Check sheet for the modelled part. Datum: model origin and axes. Units: mm. Face numbers are marked on the shaded views. A direction names the side the tool comes from. Coordinates: 2 decimals unless noted, no trailing zeros. Write each loop counter-clockwise with the first axis right and the second up, starting at its lowest first coordinate (ties: lowest second). Pieces come first, ordered by that corner, then holes. Notation, with made-up numbers: (-1, 5) -> (27, 5) arc R35 ccw to (27, 39) -> close; hole circle Ø9 at (13.25, 87). An arc over 180 degrees is marked (long way). Put each result on its own line as item: value.
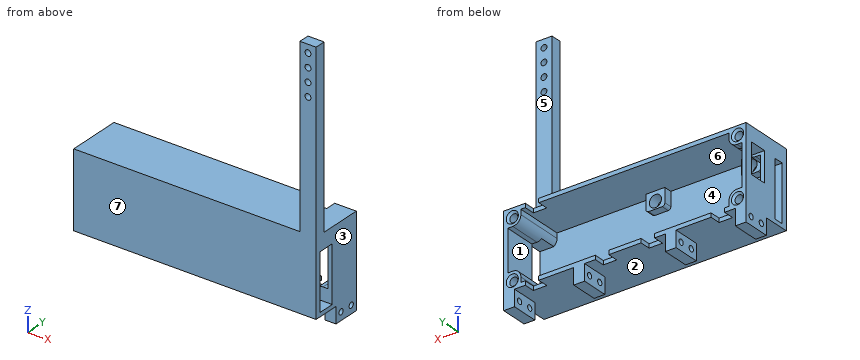
```python
from build123d import *

# Parameters (mm, degrees)
SKETCH2_W           = 87
SKETCH2_H           = 25
BOSS_EXTRUDE1_DEPTH = 2
SKETCH2_3_W         = 90
SKETCH2_3_H         = 28
SKETCH2_3_W_2       = 87
SKETCH2_3_H_2       = 25
BOSS_EXTRUDE2_DEPTH = 20
SKETCH3_W           = 4
SKETCH3_H           = 10.1
BOSS_EXTRUDE3_DEPTH = 6
SKETCH5_R           = 1.05
CUT_EXTRUDE2_DEPTH  = 105
SKETCH3_5_W         = 5
SKETCH3_5_H         = 4
CUT_EXTRUDE3_DEPTH  = 16
SKETCH2_4_W         = 6
SKETCH2_4_H         = 55
BOSS_EXTRUDE4_DEPTH = 4
SKETCH8_W           = 4.863961031
SKETCH8_H           = 4.863961031
SKETCH8_W_2         = 4.86396103
BOSS_EXTRUDE5_DEPTH = 18
SKETCH9_R           = 1.5
CUT_EXTRUDE6_DEPTH  = 5
SKETCH6_W           = 11.14966652
SKETCH6_H           = 6.5
CUT_EXTRUDE4_DEPTH  = 16
FILLET1_R           = 3
SKETCH10_W          = 20.745878282
SKETCH10_H          = 3.532229036
CUT_EXTRUDE7_DEPTH  = 109.1
SKETCH11_W          = 5
SKETCH11_H          = 4
CUT_EXTRUDE8_DEPTH  = 4
SKETCH12_W          = 20.745878282
SKETCH12_H          = 2.501759487
CUT_EXTRUDE10_DEPTH = 8
SKETCH13_R          = 2.25
BOSS_EXTRUDE6_DEPTH = 3
CHAMFER1_SIZE       = 0.75
SKETCH17_W          = 6
SKETCH17_H          = 4
BOSS_EXTRUDE9_DEPTH = 10
SKETCH7_R           = 1.1
CUT_EXTRUDE5_DEPTH  = 10
CUT_EXTRUDE11_START = -1
SKETCH18_R          = 2.25
CUT_EXTRUDE11_DEPTH = 1


with BuildPart() as part:
    # Sketch2 → Boss-Extrude1 (new body)
    with BuildSketch(Plane(origin=(0, 0, 0), x_dir=(1, 0, 0), z_dir=(0, 1, 0))):
        with Locations((-2.329700272, 12.5)):
            Rectangle(SKETCH2_W, SKETCH2_H)
    extrude(amount=BOSS_EXTRUDE1_DEPTH)

    # Sketch2<3> → Boss-Extrude2 (add)
    with BuildSketch(Plane(origin=(0, 0, 0), x_dir=(1, 0, 0), z_dir=(0, 1, 0))):
        with Locations((-2.329700272, 12.5)):
            Rectangle(SKETCH2_3_W, SKETCH2_3_H)
        with Locations((-2.329700272, 12.5)):
            Rectangle(SKETCH2_3_W_2, SKETCH2_3_H_2, mode=Mode.SUBTRACT)
    extrude(amount=BOSS_EXTRUDE2_DEPTH)

    # Sketch3 → Boss-Extrude3 (add)
    with BuildSketch(Plane(origin=(0, 0, -26.5), x_dir=(-1, 0, 0), z_dir=(0, 0, -1))):
        with Locations((45.329700272, 14.95)):
            Rectangle(SKETCH3_W, SKETCH3_H)
        with Locations((-14.670299728, 14.95)):
            Rectangle(SKETCH3_W, SKETCH3_H)
        with Locations((-40.670299728, 14.95)):
            Rectangle(SKETCH3_W, SKETCH3_H)
        with Locations((19.329700272, 14.95)):
            Rectangle(SKETCH3_W, SKETCH3_H)
    extrude(amount=BOSS_EXTRUDE3_DEPTH)

    # Sketch5 → Cut-Extrude2 (cut)
    with BuildSketch(Plane.ZY.offset(47.329700272)):
        with Locations((-29.5, 12.425)):
            Circle(SKETCH5_R)
        with Locations((-29.5, 17.475)):
            Circle(SKETCH5_R)
    extrude(amount=-CUT_EXTRUDE2_DEPTH, mode=Mode.SUBTRACT)

    # Sketch3<5> → Cut-Extrude3 (cut)
    with BuildSketch(Plane(origin=(0, 0, -26.5), x_dir=(-1, 0, 0), z_dir=(0, 0, -1))):
        with Locations((36.829700272, 18)):
            Rectangle(SKETCH3_5_W, SKETCH3_5_H)
        with Locations((10.829700272, 18)):
            Rectangle(SKETCH3_5_W, SKETCH3_5_H)
        with Locations((-32.170299728, 18)):
            Rectangle(SKETCH3_5_W, SKETCH3_5_H)
        with Locations((-6.170299728, 18)):
            Rectangle(SKETCH3_5_W, SKETCH3_5_H)
    extrude(amount=-CUT_EXTRUDE3_DEPTH, mode=Mode.SUBTRACT)

    # Sketch2<4> → Boss-Extrude4 (add)
    with BuildSketch(Plane(origin=(0, 0, 0), x_dir=(1, 0, 0), z_dir=(0, 1, 0))):
        with Locations((39.670299728, -29)):
            Rectangle(SKETCH2_4_W, SKETCH2_4_H)
    extrude(amount=BOSS_EXTRUDE4_DEPTH)

    # Sketch8 → Boss-Extrude5 (add)
    with BuildSketch(Plane(origin=(0, 2, 0), x_dir=(1, 0, 0), z_dir=(0, 1, 0))):
        with Locations((38.738319213, 22.568019484)):
            Rectangle(SKETCH8_W, SKETCH8_H)
        with Locations((38.738319213, 2.431980516)):
            Rectangle(SKETCH8_W, SKETCH8_H)
        with Locations((-43.397719757, 22.568019484)):
            Rectangle(SKETCH8_W_2, SKETCH8_H)
        with Locations((-43.397719757, 2.431980516)):
            Rectangle(SKETCH8_W_2, SKETCH8_H)
    extrude(amount=BOSS_EXTRUDE5_DEPTH)

    # Sketch9 → Cut-Extrude6 (cut)
    with BuildSketch(Plane(origin=(0, 20, 0), x_dir=(1, 0, 0), z_dir=(0, 1, 0))):
        with Locations(Location((-44.147719757, 23.318019485, 0), (0, 0, 270))):
            Circle(SKETCH9_R)
        with Locations(Location((-44.147719757, 1.681980515, 0), (0, 0, 90))):
            Circle(SKETCH9_R)
        with Locations(Location((39.488319212, 1.681980515, 0), (0, 0, 270))):
            Circle(SKETCH9_R)
        with Locations(Location((39.488319212, 23.318019485, 0), (0, 0, 90))):
            Circle(SKETCH9_R)
    extrude(amount=-CUT_EXTRUDE6_DEPTH, mode=Mode.SUBTRACT)

    # Sketch6 → Cut-Extrude4 (cut)
    with BuildSketch(Plane.ZY.offset(47.329700272)):
        with Locations((-9.5, 14)):
            Rectangle(SKETCH6_W, SKETCH6_H)
    extrude(amount=-CUT_EXTRUDE4_DEPTH, mode=Mode.SUBTRACT)

    # Fillet1
    # the kernel refuses this fillet: 3 mm, written as the material it takes off along each edge
    with BuildSketch(Plane(origin=(36.306338697, 2, -4.863961031), x_dir=(0, 0, 1), z_dir=(0, 1, 0)), Plane(origin=(-40.965739242, 2, -20.136038969), x_dir=(0, 0, -1), z_dir=(0, 1, 0))) as fillet1_piece_1:
        with BuildLine():
            CenterArc((FILLET1_R, FILLET1_R), FILLET1_R, 180, 90)
            Line((0, FILLET1_R), (0, 0))
            Line((0, 0), (FILLET1_R, 0))
        make_face()
    extrude(amount=25.5, mode=Mode.SUBTRACT)
    with BuildSketch(Plane(origin=(36.306338697, 2, -20.136038969), x_dir=(0, 0, -1), z_dir=(0, 1, 0))) as fillet1_piece_2:
        with BuildLine():
            CenterArc((FILLET1_R, -FILLET1_R), FILLET1_R, 90, 90)
            Line((0, -FILLET1_R), (0, 0))
            Line((0, 0), (FILLET1_R, 0))
        make_face()
    extrude(amount=25.5, mode=Mode.SUBTRACT)
    with BuildSketch(Plane(origin=(-40.965739242, 2, -4.863961031), x_dir=(0, 0, 1), z_dir=(0, 1, 0))) as fillet1_piece_3:
        with BuildLine():
            CenterArc((FILLET1_R, -FILLET1_R), FILLET1_R, 90, 90)
            Line((0, -FILLET1_R), (0, 0))
            Line((0, 0), (FILLET1_R, 0))
        make_face()
    extrude(amount=16.25, mode=Mode.SUBTRACT)
    with BuildSketch(Plane(origin=(-40.965739242, 9.75, -4.863961031), x_dir=(-1, 0, 0), z_dir=(0, 1, 0))) as fillet1_piece_4:
        with BuildLine():
            CenterArc((FILLET1_R, FILLET1_R), FILLET1_R, 180, 90)
            Line((0, FILLET1_R), (0, 0))
            Line((0, 0), (FILLET1_R, 0))
        make_face()
    extrude(amount=17.75, mode=Mode.SUBTRACT)

    # Sketch10 → Cut-Extrude7 (cut)
    with BuildSketch(Plane.ZY.offset(47.329700272)):
        with Locations((-14.627060859, 3.766114518)):
            Rectangle(SKETCH10_W, SKETCH10_H)
    extrude(amount=-CUT_EXTRUDE7_DEPTH, mode=Mode.SUBTRACT)

    # Sketch11 → Cut-Extrude8 (cut)
    with BuildSketch(Plane.XY.offset(1.5)):
        with Locations((32.170299728, 18)):
            Rectangle(SKETCH11_W, SKETCH11_H)
    extrude(amount=-CUT_EXTRUDE8_DEPTH, mode=Mode.SUBTRACT)

    # Sketch12 → Cut-Extrude10 (cut)
    with BuildSketch(Plane(origin=(42.670299728, 0, 0), x_dir=(0, 0, -1), z_dir=(1, 0, 0))):
        with Locations((14.627060859, 6.78310878)):
            Rectangle(SKETCH12_W, SKETCH12_H)
    extrude(amount=-CUT_EXTRUDE10_DEPTH, mode=Mode.SUBTRACT)

    # Sketch13 → Boss-Extrude6 (add)
    # profile 1 of 2: a face of its own
    with BuildSketch(Plane(origin=(0, 2, 0), x_dir=(1, 0, 0), z_dir=(0, 1, 0))):
        with BuildLine():
            Line((-40.965739242, 1.863961031), (-40.965739242, 0))
            Line((-40.965739242, 0), (-34.465739242, 0))
            Line((-34.465739242, 0), (-34.465739242, 5.247890406))
            ThreePointArc((-34.465739242, 5.247890406), (-34.758632461, 5.954997187), (-35.465739242, 6.247890406))
            Line((-35.465739242, 6.247890406), (-40.619194745, 6.247890406))
            ThreePointArc((-40.619194745, 6.247890406), (-41.102765854, 6.123195485), (-41.465739242, 5.78020837))
            ThreePointArc((-41.465739242, 5.78020837), (-41.553823791, 5.60351457), (-41.605476886, 5.412958687))
            Line((-41.605476886, 5.412958687), (-41.844418898, 3.985281374))
            ThreePointArc((-41.844418898, 3.985281374), (-41.194100644, 3.012011328), (-40.965739242, 1.863961031))
        make_face()
        with Locations(Location((-37.965739242, 3.5, 0), (0, 0, 270))):
            Circle(SKETCH13_R, mode=Mode.SUBTRACT)
    # profile 2 of 2: a face of its own
    with BuildSketch(Plane(origin=(0, 2, 0), x_dir=(1, 0, 0), z_dir=(0, 1, 0))):
        with BuildLine():
            Line((-5.965739242, 0), (1.034260758, 0))
            Line((1.034260758, 0), (1.034260758, 5.247890406))
            ThreePointArc((1.034260758, 5.247890406), (0.741367539, 5.954997187), (0.034260758, 6.247890406))
            Line((0.034260758, 6.247890406), (-4.965739242, 6.247890406))
            ThreePointArc((-4.965739242, 6.247890406), (-5.672846023, 5.954997187), (-5.965739242, 5.247890406))
            Line((-5.965739242, 5.247890406), (-5.965739242, 0))
        make_face()
        with Locations(Location((-2.465739242, 3.5, 0), (0, 0, 270))):
            Circle(SKETCH13_R, mode=Mode.SUBTRACT)
    extrude(amount=BOSS_EXTRUDE6_DEPTH)

    # Chamfer1
    chamfer1_edges = [part.edges().sort_by_distance(p)[0] for p in [
        (39.488319212, 20, -21.818019485),
        (39.488319212, 20, -3.181980515),
        (-44.147719757, 20, -0.181980515),
        (-44.147719757, 20, -24.818019485),
    ]]
    chamfer(chamfer1_edges, length=CHAMFER1_SIZE)

    # Sketch17 → Boss-Extrude9 (add)
    with BuildSketch(Plane.XY.offset(56.5)):
        with Locations((39.670299728, 2)):
            Rectangle(SKETCH17_W, SKETCH17_H)
    extrude(amount=BOSS_EXTRUDE9_DEPTH)

    # Sketch7 → Cut-Extrude5 (cut)
    with BuildSketch(Plane(origin=(0, 4, 0), x_dir=(1, 0, 0), z_dir=(0, 1, 0))):
        with Locations(Location((39.670299728, -63.5, 0), (0, 0, 270))):
            Circle(SKETCH7_R)
        with Locations(Location((39.670299728, -58.5, 0), (0, 0, 270))):
            Circle(SKETCH7_R)
        with Locations(Location((39.670299728, -48.5, 0), (0, 0, 270))):
            Circle(SKETCH7_R)
        with Locations(Location((39.670299728, -53.5, 0), (0, 0, 270))):
            Circle(SKETCH7_R)
    extrude(amount=-CUT_EXTRUDE5_DEPTH, mode=Mode.SUBTRACT)

    # Sketch18 → Cut-Extrude11 (cut)
    with BuildSketch(Plane(origin=(0, 2, 0), x_dir=(1, 0, 0), z_dir=(0, 1, 0)).offset(CUT_EXTRUDE11_START)):
        with Locations(Location((-37.965739242, 3.5, 0), (0, 0, 270))):
            Circle(SKETCH18_R)
        with Locations(Location((-2.465739242, 3.5, 0), (0, 0, 270))):
            Circle(SKETCH18_R)
    extrude(amount=CUT_EXTRUDE11_DEPTH, mode=Mode.SUBTRACT)


solid = part.part
```
Q1. Mould release check, pull along Z, two halves, no side actions. Record for the marked faces 1, 2, 3 and 4: released by +Z, released by -Z, zero draft, split by the parting line, or undercut.
Recorded:
face 1: undercut
face 2: released by -Z
face 3: zero draft
face 4: undercut
Q2. Cross-section at C-C (z = 22). Record the cut outline in (x, y).
Recorded:
outline: (36.67, 0) -> (42.67, 0) -> (42.67, 4) -> (36.67, 4) -> close
Q3. Tool access check on the marked faces 5, 6 and 7. Record the directions out of +Z, -Z, +X, -X, +Y, -Y that give a thin tool (end or side, any length) a straight path to the whole face; none if there is none.
Recorded:
face 5: +Z, +X, -X, +Y
face 6: +Y
face 7: +Z, -Z, +X, -X, -Y
Q4. Cross-section at B-B (x = 31). Record the cut outline in (y, z).
Recorded:
outline: (0, -26.5) -> (16, -26.5) -> (16, -25) -> (2, -25) -> (2, 0) -> (16, 0) -> (16, 1.5) -> (0, 1.5) -> close
Q5. Depth check by flat-ended pin: P1, Ø3, axis at x = 2.5, y = 11, coming from the -Z side; P2, Ø3.5, axis at x = -38.5, z = -2.5, coming from the +Y side; P3, Ø2, axis at x = -20.5, y = 13.5, coming from the +Z side. Enter the tip coordinate at first touch or a pass-through.
Recorded:
P1: stops at z = -26.5
P2: stops at y = 5
P3: stops at z = 1.5
Q6. Cross-section at A-A (z = 63.5). Record the cut outline in (x, y).
Recorded:
outline: (36.67, 0) -> (38.57, 0) -> (38.57, 4) -> (36.67, 4) -> close; (40.77, 0) -> (42.67, 0) -> (42.67, 4) -> (40.77, 4) -> close
Q7. Material ranges on line 1 along Z through (x, y) = (-1, 6.25); line 2 along Z through (x, y) = (-19.5, 17.75); line 3 along X through (y, z) = (3.95, -3.5), recorded low to high.
Recorded:
line 1: z = -26.5 to -25, 0 to 1.5
line 2: z = -32.5 to -30.51, -28.49 to -25, 0 to 1.5
line 3: x = -47.33 to -40.22, -35.72 to -34.47, -5.97 to -4.72, -0.22 to 1.03, 36.79 to 42.67
